For this review, take the finished solid that the model builds, in its own axes (mm). A direction names the side the tool comes from. Give positions to 0.01 mm unless a question says otherwise; leave off trailing zeros. Order: outer loops, then holes, each group sorted by start corner. A loop starts at its lowest first (then second) coordinate and runs counter-clockwise, first axis right, second up.
Autodesk Inventor part; units mm, degrees
ref_plane "rot_XY" through (0, 6.6675, 0) normal (1, 0, 0) x (0, 0, -1)
ref_plane "rot_YZ" through (0, 6.6675, 0) normal (0, 0, -1) x (0, 1, 0)
ref_plane "rot_ZX" through (0, 6.6675, 0) normal (0, 1, 0) x (1, 0, 0)
sketch "Sketch_2" plane through (0, -0.254, 0) normal (0, 1, 0) x (1, 0, 0)
  line L0 (-3.9497, -5.1435) -> (-3.9497, -6.3724)
  arc A0 (-3.9497, -6.3724) -> (-3.8197, -6.5024) centre (-3.8197, -6.3724) ccw
  line L1 (-3.8197, -6.5024) -> (3.8197, -6.5024)
  arc A1 (3.8197, -6.5024) -> (3.9497, -6.3724) centre (3.8197, -6.3724) ccw
  line L2 (3.9497, -6.3724) -> (3.9497, -5.1435)
  line L3 (3.9497, -5.1435) -> (3.6957, -5.1435)
  line L4 (3.6957, -5.1435) -> (3.6957, -2.9397)
  line L5 (3.6957, -2.9397) -> (3.3147, -2.8725)
  line L6 (3.3147, -2.8725) -> (3.3147, -1.8265)
  line L7 (3.3147, -1.8265) -> (3.6957, -1.7593)
  line L8 (3.6957, -1.7593) -> (3.6957, 1.7593)
  line L9 (3.6957, 1.7593) -> (3.3147, 1.8265)
  line L10 (3.3147, 1.8265) -> (3.3147, 2.8725)
  line L11 (3.3147, 2.8725) -> (3.6957, 2.9397)
  line L12 (3.6957, 2.9397) -> (3.6957, 5.1435)
  line L13 (3.6957, 5.1435) -> (3.9497, 5.1435)
  line L14 (3.9497, 5.1435) -> (3.9497, 6.3724)
  arc A2 (3.9497, 6.3724) -> (3.8197, 6.5024) centre (3.8197, 6.3724) ccw
  line L15 (3.8197, 6.5024) -> (-3.8197, 6.5024)
  arc A3 (-3.8197, 6.5024) -> (-3.9497, 6.3724) centre (-3.8197, 6.3724) ccw
  line L16 (-3.9497, 6.3724) -> (-3.9497, 5.1435)
  line L17 (-3.9497, 5.1435) -> (-3.6957, 5.1435)
  line L18 (-3.6957, 5.1435) -> (-3.6957, 2.9397)
  line L19 (-3.6957, 2.9397) -> (-3.3147, 2.8725)
  line L20 (-3.3147, 2.8725) -> (-3.3147, 1.8265)
  line L21 (-3.3147, 1.8265) -> (-3.6957, 1.7593)
  line L22 (-3.6957, 1.7593) -> (-3.6957, -1.7593)
  line L23 (-3.6957, -1.7593) -> (-3.3147, -1.8265)
  line L24 (-3.3147, -1.8265) -> (-3.3147, -2.8725)
  line L25 (-3.3147, -2.8725) -> (-3.6957, -2.9397)
  line L26 (-3.6957, -2.9397) -> (-3.6957, -5.1435)
  line L27 (-3.6957, -5.1435) -> (-3.9497, -5.1435)
extrude "Extrusion1" add sketch "Sketch_2" against normal blind 9.1694
sketch "Sketch_1" plane through (0, -9.4234, 0) normal (0, 1, 0) x (1, 0, 0)
  line L0 (-3.1877, 6.1184) -> (-3.1877, -6.1184)
  arc A0 (-3.1877, -6.1184) -> (-3.0577, -6.2484) centre (-3.0577, -6.1184) ccw
  line L1 (-3.0577, -6.2484) -> (3.0577, -6.2484)
  arc A1 (3.0577, -6.2484) -> (3.1877, -6.1184) centre (3.0577, -6.1184) ccw
  line L2 (3.1877, -6.1184) -> (3.1877, 6.1184)
  arc A2 (3.1877, 6.1184) -> (3.0577, 6.2484) centre (3.0577, 6.1184) ccw
  line L3 (3.0577, 6.2484) -> (-3.0577, 6.2484)
  arc A3 (-3.0577, 6.2484) -> (-3.1877, 6.1184) centre (-3.0577, 6.1184) ccw
extrude "Extrusion2" cut sketch "Sketch_1" along normal blind 0.0254
sketch "Sketch_7" plane through (0, -9.4234, 0) normal (0, 1, 0) x (1, 0, 0)
  line L0 (-1.0033, 5.0927) -> (-1.0033, 4.3053)
  line L1 (-1.0033, 4.3053) -> (1.0033, 4.3053)
  line L2 (1.0033, 4.3053) -> (1.0033, 5.0927)
  line L3 (1.0033, 5.0927) -> (-1.0033, 5.0927)
extrude "Extrusion3" cut sketch "Sketch_7" along normal blind 0.254
pattern_linear "Rectangular Pattern1" count 2 spacing 4.699 along (0, 0, 1) of "Extrusion3"
ref_plane "rot_XY" through (0, 6.6675, 0) normal (1, 0, 0) x (0, 0, -1)
ref_plane "rot_YZ" through (0, 6.6675, 0) normal (0, 0, -1) x (0, 1, 0)
ref_plane "rot_ZX" through (0, 6.6675, 0) normal (0, 1, 0) x (1, 0, 0)
ref_plane "to_cover_XY" through (0, -0.254, 0) normal (0, 1, 0) x (1, 0, 0)
ref_plane "to_cover_YZ" through (0, -0.254, 0) normal (1, 0, 0) x (0, 0, -1)
ref_plane "to_cover_ZX" through (0, -0.254, 0) normal (0, 0, -1) x (0, 1, 0)
ref_plane "to_terminals_XY" through (0, -9.4234, 0) normal (0, 1, 0) x (1, 0, 0)
ref_plane "to_terminals_YZ" through (0, -9.4234, 0) normal (1, 0, 0) x (0, 0, -1)
ref_plane "to_terminals_ZX" through (0, -9.4234, 0) normal (0, 0, -1) x (0, 1, 0)
properties part number "M20111SS1W01-switch"
1) We need section A-A on x = 3.5. Give the boundary of the cut face in (y, z), then the cut area to 3 significant figures.
Answer sheet:
outline: (-9.42, -6.5) - (-0.25, -6.5) - (-0.25, -2.91) - (-9.42, -2.91) - close; (-9.42, -1.79) - (-0.25, -1.79) - (-0.25, 1.79) - (-9.42, 1.79) - close; (-9.42, 2.91) - (-0.25, 2.91) - (-0.25, 6.5) - (-9.42, 6.5) - close
area: 98.9 mm2
2) To check wall thickness, follow line 1 (X direction, y = -5.25, z = -4.75); line 2 (Y direction, x = -2, z = -5.5); line 3 (X direction, y = -3, z = 2). State the ranges of each line that lie inside material, in increasing order.
Answer sheet:
line 1: x = -3.7 to 3.7
line 2: y = -9.4 to -0.25
line 3: x = -3.31 to 3.31
3) Clearance check with flat-ended pins moving along their axes: pin 1 (2.5 mm diameter, centred on y = -5, z = -3.5, fed in from +X); pin 2 (1 mm diameter, centred on x = -1, z = 0, fed in from -Y); pin 3 (1.1 mm diameter, centred on y = -6, z = -0.5, fed in from -X). State where each tip first meets the part, or that it passes through.
Answer sheet:
pin 1: stops at x = 3.7
pin 2: stops at y = -9.4
pin 3: stops at x = -3.7
4) Draft analysis for pull direction Z (two halves, no side actions). For faces 1 (the face through (3.696, -5, 0)), 2 (the face through (0, -5, -6.502)), 3 (the face through (-3.95, -5, -6)), state which applies: +Z half, -Z half, draft (parallel to the pull), parting line (faces both ways), or undercut.
Answer sheet:
face 1: undercut
face 2: -Z half
face 3: draft
5) Tool access review of faces 4 (the face through (3.315, -5, 2)), 5 (the face through (0, -9.398, -1)), 6 (the face through (-3.315, -5, 2)), 7 (the face through (3.95, -5, 6)): name each direction out of +Z, -Z, +X, -X, +Y, -Y from which nothing blocks a thin tool from reaching the whole face with its end or side.
Answer sheet:
face 4: +X, +Y, -Y
face 5: -Y
face 6: -X, +Y, -Y
face 7: +Z, -Z, +X, +Y, -Y
